Here's how the part is built. I have some questions about the finished solid (model axes, mm). A direction names the side the tool comes from. Give positions to 0.01 mm unless a question says otherwise; leave off trailing zeros. Write each loop counter-clockwise with the first axis right and the second up, starting at its lowest first coordinate (ties: lowest second). Pieces come first, ordered by that corner, then holes. Notation, with made-up numbers: (-23.75, 84) -> (14.25, 84) arc R29 cw to (14.25, 117) -> close; hole circle Ø8 at (80.25, 35.5). An arc over 180 degrees is marked (long way). Use CSV: the item, a comma, the result in double quotes. Start each with the question number.
(1) Which directions (+Z, -Z, +X, -X, +Y, -Y) give clear straight access to the entire face, cutting with the end or side of a thin tool? Please do faces 4 (the cylindrical face through (-4.13, -20.67, 14.35)), 5 (the flat face through (265, 35, -9)), 6 (the flat face through (-280, 20.156, -30)).
(2) For pin 1 Ø6 at (x, z) = (219.5, -15) entering from +Y; pin 2 Ø1.5 at (x, y) = (-144.5, -5) entering from -Z; pin 3 Ø4 at (x, y) = (43.5, 10.5) entering from +Z, each with a flat end and sliding along its axis, tell me the tip position at first contact or that it passes through.
(3) Suppose I cut it at C-C on x = -235.5. List the corners of the cut face in (y, z) for me, plus the area to 3 significant figures.
(4) Suppose I cut it at B-B on z = -36. List the corners of the cut face in (x, y) for me, plus the area to 3 significant figures.
(5) If we mould it in two halves opening along X, with no side actions, what happens to faces 1 (the flat face through (280, 20.156, -29)), 2 (the flat face through (303.66, 21, 3)), 3 (the flat face through (-265, 35, -10))? For each: pulls with the +X half, pulls with the -X half, needs draft (parallel to the pull), parting line crosses it, or undercut.
(6) Suppose I cut it at A-A on y = 36. List the corners of the cut face in (x, z) for me.
(7) Suppose I cut it at D-D on z = 2. List the corners of the cut face in (x, y) for me, plus the area to 3 significant figures.
(8) I need wall thicknesses on L1, parallel to X at y = 38, z = -23.5; L2, parallel to X at y = 23, z = 10.5; L3, parallel to X at y = 39, z = 13. Which ranges of each line are inside material? Lowest first, please. Write a range as [from, to].
Autodesk Inventor part; units mm, degrees
ref_plane "YZ Plane" through (0, 0, 0) normal (1, 0, 0) x (0, 1, 0)
ref_plane "XZ Plane" through (0, 0, 0) normal (0, 1, 0) x (-1, 0, 0)
ref_plane "XY Plane" through (0, 0, 0) normal (0, 0, 1) x (1, 0, 0)
sketch "Эскиз1" plane through (0, 0, 0) normal (1, 0, 0) x (0, 1, 0)
  line L0 (20.1556, 25.3526) -> (20.1556, -14.6474)
  line L1 (20.1556, -14.6474) -> (-49.8444, -14.6474)
  arc A0 (20.1556, 25.3526) -> (-49.8444, -14.6474) centre (20.1556, -55.8974) ccw
  line L2 (20.1556, -14.6474) -> (-20.1556, 14.6474) construction
  point P0 (0, 0)
  point P1 (0, 0)
  dimension "d0" = 70
  dimension "d2" = 40
extrude "Выдавливание1" add sketch "Эскиз1" along normal mid plane 590
sketch "Эскиз6" plane through (295, 0, 0) normal (1, 0, 0) x (0, 0, -1)
  line L0 (14.6474, 20.1556) -> (-25.3526, 20.1556)
  line L1 (-25.3526, 20.1556) -> (44.6474, 20.1556)
  line L2 (44.6474, 20.1556) -> (44.6474, 50.1556)
  line L3 (44.6474, 50.1556) -> (-25.3526, 50.1556)
  line L4 (-25.3526, 50.1556) -> (-25.3526, 20.1556)
  point P0 (0, 0)
  dimension "d13" = 70
  dimension "d14" = 30
extrude "Выдавливание3" add sketch "Эскиз6" against normal blind 30
sketch "Эскиз7" plane through (295, 50.1556, 25.3526) normal (0, 1, 0) x (1, 0, 0)
  line L0 (0, 29.5) -> (8.6603, 34.5)
  line L1 (0, 14.5) -> (0, 29.5)
  line L2 (8.6603, 9.5) -> (0, 14.5)
  line L3 (8.6603, 34.5) -> (8.6603, 9.5)
  point P0 (-295, 25.3526)
extrude "Выдавливание4" add sketch "Эскиз7" against normal blind 60
mirror "Зеркальное отражение3" about plane through (0, 0, 0) normal (1, 0, 0) of "Выдавливание3", "Выдавливание4"
properties part number "Нижний край"
Geometry says:
1,face 4,"+Z, +X, -X, -Y"
1,face 5,"+Z, -Z, +Y"
1,face 6,"-Z, +X, -X, -Y"
2,pin 1,"y = 20.16"
2,pin 2,"z = -14.65"
2,pin 3,"z = 24.99"
3,outline,"(-49.84, -14.65) -> (20.16, -14.65) -> (20.16, 25.35) arc R81.25 ccw to start"
3,area,"1,980 mm²"
4,outline,"(-295, 20.16) -> (-265, 20.16) -> (-265, 50.16) -> (-295, 50.16) -> close; (265, 20.16) -> (295, 20.16) -> (295, 50.16) -> (265, 50.16) -> close"
4,area,"1,800 mm²"
5,face 1,"needs draft"
5,face 2,"pulls with the +X half"
5,face 3,"undercut"
6,outline,"(-303.66, -9.15) -> (-295, -4.15) -> (-295, -44.65) -> (-265, -44.65) -> (-265, 25.35) -> (-295, 25.35) -> (-295, 10.85) -> (-303.66, 15.85) -> close; (265, -44.65) -> (295, -44.65) -> (295, -4.15) -> (303.66, -9.15) -> (303.66, 15.85) -> (295, 10.85) -> (295, 25.35) -> (265, 25.35) -> close"
7,outline,"(-303.66, -9.84) -> (-295, -9.84) -> (-295, -36.85) -> (295, -36.85) -> (295, -9.84) -> (303.66, -9.84) -> (303.66, 50.16) -> (265, 50.16) -> (265, 20.16) -> (-265, 20.16) -> (-265, 50.16) -> (-303.66, 50.16) -> close"
7,area,"36,500 mm²"
8,L1,"[-295, -265], [265, 295]"
8,L2,"[-303.66, -265], [265, 303.66]"
8,L3,"[-303.66, -298.72], [-295, -265], [265, 295], [298.72, 303.66]"
